from build123d import *

# Parameters (mm, degrees)
BOSS_EXTRUDE1_DEPTH                        = 150
CUT_EXTRUDE1_DEPTH                         = 227.715680975
CUT_EXTRUDE1_DEPTH_BACK                    = 227.715680975
SKETCH3_W                                  = 170
SKETCH3_H                                  = 190
CUT_EXTRUDE2_DEPTH                         = 70
CUT_EXTRUDE3_DEPTH                         = 100
CUT_EXTRUDE3_DRAFT                         = -18.43
SKETCH7_R                                  = 5
CUT_EXTRUDE5_DEPTH                         = 266.706605112
SKETCH9_W                                  = 10
SKETCH9_H                                  = 3
SKETCH9_W_2                                = 5
SKETCH9_H_2                                = 15
BOSS_EXTRUDE2_DEPTH                        = 15
SKETCH10_R                                 = 8
CUT_EXTRUDE6_DEPTH                         = 40
MIRROR1_AT_THE_SECOND_PLANE_COPY_1_SKETC_R = 8
MIRROR1_AT_THE_SECOND_PLANE_COPY_1_DEPTH   = 40


with BuildPart() as part:
    # Sketch1 → Boss-Extrude1 (new body)
    with BuildSketch(Plane(origin=(0, 0, 0), x_dir=(1, 0, 0), z_dir=(0, 1, 0))):
        Polygon((-150, 30), (-100, 80), (100, 80), (150, 30), (150, -30), (100, -80), (-100, -80), (-150, -30), align=None)
    extrude(amount=BOSS_EXTRUDE1_DEPTH)

    # Sketch2 → Cut-Extrude1 (cut, two sides: drawn at the far end of the back side and taken through both)
    with BuildSketch(Plane.XY.offset(-CUT_EXTRUDE1_DEPTH_BACK)):
        Polygon((-150, 150), (-100, 0), (-150, 0), align=None)
        Polygon((100, 0), (150, 150), (150, 0), align=None)
    extrude(amount=CUT_EXTRUDE1_DEPTH + CUT_EXTRUDE1_DEPTH_BACK, mode=Mode.SUBTRACT)

    # Sketch3 → Cut-Extrude2 (cut, symmetric)
    with BuildSketch(Plane.XY):
        with Locations((0, 105)):
            Rectangle(SKETCH3_W, SKETCH3_H)
    extrude(amount=CUT_EXTRUDE2_DEPTH, both=True, mode=Mode.SUBTRACT)


with BuildPart() as cut_extrude3_tool:
    # Sketch4 → Cut-Extrude3 (with draft: the straight prism first)
    with BuildSketch(Plane(origin=(0, 150, 0), x_dir=(1, 0, 0), z_dir=(0, 1, 0))):
        Polygon((-140, -25), (-125, -40), (-95, -70), (95, -70), (140, -25), (140, 25), (95, 70), (-95, 70), (-140, 25), align=None)
    extrude(amount=-CUT_EXTRUDE3_DEPTH)
    # Cut-Extrude3: the draft: its side faces are tilted about the plane it starts from
    cut_extrude3_sides = [cut_extrude3_tool.faces().sort_by_distance(p)[0] for p in [
        (-117.5, 100, 47.5),
        (-117.5, 100, -47.5),
        (0, 100, -70),
        (117.5, 100, -47.5),
        (140, 100, 0),
        (117.5, 100, 47.5),
        (0, 100, 70),
        (-140, 100, 0),
    ]]
    draft(cut_extrude3_sides, Plane(origin=(0, 150, 0), x_dir=(1, 0, 0), z_dir=(0, 1, 0)), CUT_EXTRUDE3_DRAFT)


with BuildPart() as part_1:
    add(part.part)

    # Cut-Extrude3: cut by cut_extrude3_tool
    add(cut_extrude3_tool.part, mode=Mode.SUBTRACT)

    # Sketch7 → Cut-Extrude5 (cut, through all)
    with BuildSketch(Plane.XY.offset(80)):
        with Locations((-60, 40)):
            Circle(SKETCH7_R)
        with Locations((60, 40)):
            Circle(SKETCH7_R)
    extrude(amount=-CUT_EXTRUDE5_DEPTH, mode=Mode.SUBTRACT)

    # Sketch9 → Boss-Extrude2 (add)
    with BuildSketch(Plane(origin=(0, 10, 0), x_dir=(1, 0, 0), z_dir=(0, 1, 0))):
        with Locations((70, 3.5)):
            Rectangle(SKETCH9_W, SKETCH9_H)
        with Locations((-22.5, -42.5)):
            Rectangle(SKETCH9_W_2, SKETCH9_H_2)
    extrude(amount=BOSS_EXTRUDE2_DEPTH)

    # Sketch10 → Cut-Extrude6 (cut)
    with BuildSketch(Plane(origin=(-42.441799319, -20.001495929, 42.441799319), x_dir=(-0.6068291050905237, -0.2859796255102719, -0.7416023806650293), z_dir=(0.670839704394397, 0.31614582397380653, -0.6708397043943964))):
        with Locations(Location((-14.755059332, 151.805613608, 0), (0, 0, 17.544132392))):
            Circle(SKETCH10_R)
        with Locations(Location((9.082066856, 159.341621508, 0), (0, 0, 17.544132392))):
            Circle(SKETCH10_R)
    cut_extrude6 = extrude(amount=-CUT_EXTRUDE6_DEPTH, mode=Mode.SUBTRACT)

    # Mirror1: Cut-Extrude6 across plane
    add(cut_extrude6.mirror(Plane(origin=(0, 0, 0), x_dir=(0, 0, 1), z_dir=(1, 0, 0))), mode=Mode.SUBTRACT)

    # Mirror1 at the second plane: Cut-Extrude6 across plane
    add(cut_extrude6.mirror(Plane.XY), mode=Mode.SUBTRACT)

    # Mirror1 at the second plane copy 1 sketc → Mirror1 at the second plane copy 1 (cut)
    with BuildSketch(Plane(origin=(42.441799319, -20.001495929, -42.441799319), x_dir=(0.6068291050905237, -0.2859796255102719, 0.7416023806650293), z_dir=(-0.670839704394397, 0.31614582397380653, 0.6708397043943964))):
        with Locations(Location((-14.755059332, 151.805613608, 0), (0, 0, 17.544132392))):
            Circle(MIRROR1_AT_THE_SECOND_PLANE_COPY_1_SKETC_R)
        with Locations(Location((9.082066856, 159.341621508, 0), (0, 0, 17.544132392))):
            Circle(MIRROR1_AT_THE_SECOND_PLANE_COPY_1_SKETC_R)
    extrude(amount=-MIRROR1_AT_THE_SECOND_PLANE_COPY_1_DEPTH, mode=Mode.SUBTRACT)


solid = part_1.part
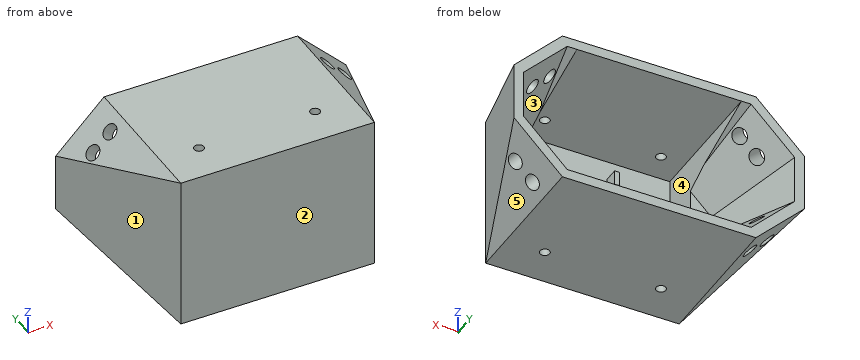
Build history of the part. All positions in model axes, mm. Face numbers are marked on the shaded views. A direction names the side the tool comes from. Coordinates: 2 decimals unless noted, no trailing zeros. Write each loop counter-clockwise with the first axis right and the second up, starting at its lowest first coordinate (ties: lowest second). Pieces come first, ordered by that corner, then holes. Notation, with made-up numbers: (-12, 23) -> (28, 23) arc R9 cw to (28, 34) -> close; hole circle Ø2 at (6, 31). An arc over 180 degrees is marked (long way). Use CSV: the item, a comma, the result in double quotes. Start each with the question number.
Q1. Cut at B-B, the plane y = 16.5. List the corners of the cut face in (x, z).
Q2. Cut at C-C, the plane z = 3.5. List the corners of the cut face in (x, y).
Q3. Pull direction X, two halves, no side cores. Call the marked faces 1, 2 and 3: released by +X, released by -X, zero draft, split by the parting line, or undercut.
Q4. Cut at D-D, the plane y = 40. List the corners of the cut face in (x, z).
Q5. Drill centre lines: probe 1 along Y at (x, z) = (60, 77.5); probe 2 along Z at (x, y) = (-13.5, 125); probe 3 along X at (y, z) = (123, 64). Where is each one in solid material? Low to high.
Q6. 3-axis set-ups, long thin cutter, end or side, ignore diameter. For the marked faces 4 and 5: which of +Z, -Z, +X, -X, +Y, -Y reach the whole face in a straight line?
Q7. Cut at A-A, the plane x = -60. List the corners of the cut face in (y, z).
Q8. Flat gauge pins, fed straight in: pin 1 Ø4 at (y, z) = (114, 60) entering from +X; pin 2 Ø1.5 at (y, z) = (14, -3) entering from -X; pin 3 Ø11 at (x, z) = (-91.5, 10.5) entering from +Y. Where does each tip first touch, or does it go through?
Checked values:
1,outline,"(-105.5, -74.5) -> (-100, -80) -> (100, -80) -> (105.5, -74.5) -> (105.5, 74.5) -> (100, 80) -> (-100, 80) -> (-105.5, 74.5) -> close; (-25, 35) -> (-20, 35) -> (-20, 50) -> (-25, 50) -> close; (65, -5) -> (75, -5) -> (75, -2) -> (65, -2) -> close; hole (-85, -70) -> (85, -70) -> (85, 70) -> (-85, 70) -> close"
2,outline,"(-150, 150) -> (-100, 0) -> (100, 0) -> (150, 150) -> (140, 150) -> (106.68, 50) -> (85, 50) -> (85, 10) -> (-85, 10) -> (-85, 50) -> (-106.68, 50) -> (-140, 150) -> close"
3,face 1,"released by -X"
3,face 2,"zero draft"
3,face 3,"undercut"
4,outline,"(-113.33, -66.67) -> (-100, -80) -> (-65, -80) -> (-65, -70) -> (-85, -70) -> (-85, 70) -> (-65, 70) -> (-65, 80) -> (-100, 80) -> (-113.33, 66.67) -> close; (-55, -80) -> (55, -80) -> (55, -70) -> (-55, -70) -> close; (-55, 70) -> (55, 70) -> (55, 80) -> (-55, 80) -> close; (65, -80) -> (100, -80) -> (113.33, -66.67) -> (113.33, 66.67) -> (100, 80) -> (65, 80) -> (65, 70) -> (85, 70) -> (85, -70) -> (65, -70) -> close"
5,probe 1,"y = 0 to 35, 45 to 150"
5,probe 2,"z = -80 to -70, 70 to 80"
5,probe 3,"x = -116 to -113.69, -98.96 to -85, 85 to 98.96, 113.69 to 116"
6,face 4,"+Y"
6,face 5,"-Z, +X, +Y, -Y"
7,outline,"(0, -80) -> (35, -80) -> (35, -70) -> (10, -70) -> (10, 70) -> (35, 70) -> (35, 80) -> (0, 80) -> close; (45, -80) -> (150, -80) -> (150, -70) -> (45, -70) -> close; (45, 70) -> (150, 70) -> (150, 80) -> (45, 80) -> close"
8,pin 1,"stops at x = 122"
8,pin 2,"stops at x = -104.92"
8,pin 3,"stops at y = 50"
